For this review, take the finished solid that the model builds, in its own axes (mm). Face numbers are marked on the shaded views. A direction names the side the tool comes from. Round coordinates to 2 decimals unless told otherwise and drop trailing zeros. Order: outer loops, then holes, each group sorted by start corner. A loop starts at its lowest first (then second) coordinate and runs counter-clockwise, first axis right, second up. Notation, with made-up numbers: M -28,30 L -22,30 A8 ccw -22,41 Z; hole C -16.5,22.5 d8. An arc over 180 degrees is marked long. Write item = value, one per line. Start each with the question number.
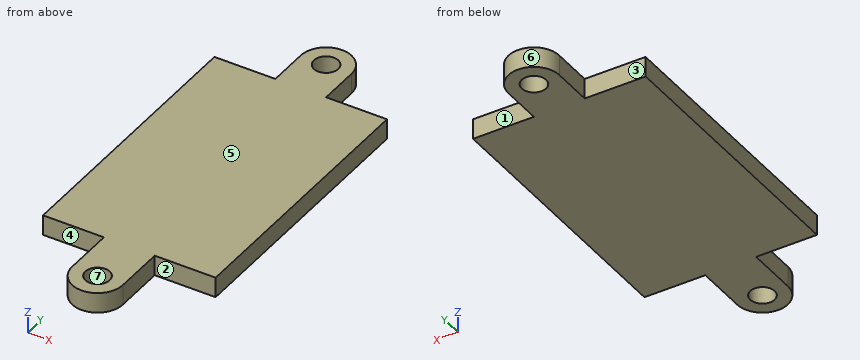
from build123d import *

# Parameters (mm, degrees)
SKETCH1_R           = 3.175
SKETCH1_R_2         = 1.524
SKETCH1_W           = 21.59
SKETCH1_H           = 34.29
BOSS_EXTRUDE1_DEPTH = 2.54


with BuildPart() as part:
    # Sketch1 → Boss-Extrude1 (new body)
    # profile 1 of 5: a face of its own
    with BuildSketch(Plane.XY):
        with Locations((10.795, 39.37)):
            Circle(SKETCH1_R)
        with Locations((10.795, 39.37)):
            Circle(SKETCH1_R_2, mode=Mode.SUBTRACT)
    # profile 2 of 5: a face of its own
    with BuildSketch(Plane.XY):
        with BuildLine():
            ThreePointArc((13.97, 39.37), (10.795, 36.195), (7.62, 39.37))
            Line((7.62, 39.37), (7.62, 34.29))
            Line((7.62, 34.29), (13.97, 34.29))
            Line((13.97, 34.29), (13.97, 39.37))
        make_face()
    # profile 3 of 5: a face of its own
    with BuildSketch(Plane.XY):
        with Locations((10.795, 17.145)):
            Rectangle(SKETCH1_W, SKETCH1_H)
    # profile 4 of 5: a face of its own
    with BuildSketch(Plane.XY):
        with BuildLine():
            Line((13.97, 0), (7.62, 0))
            Line((7.62, 0), (7.62, -6.35))
            ThreePointArc((7.62, -6.35), (10.795, -3.175), (13.97, -6.35))
            Line((13.97, -6.35), (13.97, 0))
        make_face()
    # profile 5 of 5: a face of its own
    with BuildSketch(Plane.XY):
        with Locations((10.795, -6.35)):
            Circle(SKETCH1_R)
        with Locations((10.795, -6.35)):
            Circle(SKETCH1_R_2, mode=Mode.SUBTRACT)
    extrude(amount=BOSS_EXTRUDE1_DEPTH)


solid = part.part
(1) Insertion check: pin 1 (1.3 mm diameter, centred on y = 36.5, z = 1, fed in from +X); pin 2 (1.3 mm diameter, centred on x = 16.5, z = 1.5, fed in from -Y); pin 3 (1.3 mm diameter, centred on x = 3, z = 1.5, fed in from +Y). Each pin has a flat end and moves straight along its axis. Give the tip position at first contact, or say it passes through.
(2) For the marked faces 1, 2, 3 and 4, list the 3-axis set-ups (+Z, -Z, +X, -X, +Y, -Y) from which the entire face can be reached by the end or side of a thin tool; tool diameter is ignored.
(3) For line 1 along Y through (x, z) = (1.75, 1.45); line 2 along Y through (x, z) = (11, 2.45); line 3 along Y through (x, z) = (10.25, 0.6), list the stretches that pass through material, from the lowest coordinate up.
(4) We need section A-A, the plane z = 1.7. Write out the cut boundary in (x, y) (3 decimals).
(5) Draft analysis for pull direction X (two halves, no side actions). For the marked faces 5, 6 and 7, state which applies: released by +X, released by -X, zero draft, split by the parting line, or undercut.
(6) We need section B-B, the plane y = -1. Write out the cut boundary in (x, z), then the cut area to 3 significant figures.
Values:
q1.pin_1 = 13.97
q1.pin_2 = 0
q1.pin_3 = 34.29
q2.face_1 = +Z, -Z, +X, +Y
q2.face_2 = +Z, -Z, +X, -Y
q2.face_3 = +Z, -Z, -X, +Y
q2.face_4 = +Z, -Z, -X, -Y
q3.line_1 = 0 to 34.29
q3.line_2 = -9.52 to -7.86, -4.84 to 37.86, 40.88 to 42.54
q3.line_3 = -9.48 to -7.77, -4.93 to 37.95, 40.79 to 42.5
q4.outline = M 0,0 L 7.62,0 L 7.62,-6.35 A3.175 ccw 13.97,-6.35 L 13.97,0 L 21.59,0 L 21.59,34.29 L 13.97,34.29 L 13.97,39.37 A3.175 ccw 7.62,39.37 L 7.62,34.29 L 0,34.29 Z; hole C 10.795,-6.35 d3.048; hole C 10.795,39.37 d3.048
q5.face_5 = zero draft
q5.face_6 = split by the parting line
q5.face_7 = undercut
q6.outline = M 7.62,0 L 13.97,0 L 13.97,2.54 L 7.62,2.54 Z
q6.area = 16.1 mm²
